```python
from build123d import *

# Parameters (mm, degrees)
SKETCH_1_R          = 2.5
EXTRUDE_1_DEPTH     = 2.5
EXTRUDE_1_2_DEPTH   = 2.5
EXTRUDE_1_3_DEPTH   = 2.5
SKETCH_2_R          = 1.5
EXTRUDE_2_DEPTH     = 2.5
SKETCH_3_W          = 5.060610533
SKETCH_3_H          = 13.613755096
EXTRUDE_3_DEPTH     = 2.5
SKETCH_4_W          = 80.650749302
SKETCH_4_H          = 55.377698756
EXTRUDE_4_DEPTH     = 2
SKETCH_5_W          = 80.650749302
SKETCH_5_H          = 55.377698756
SKETCH_5_W_2        = 75.650749302
SKETCH_5_H_2        = 50.377698756
EXTRUDE_5_DEPTH     = 13
FILLET_1_R          = 2.5
CUT_EXTRUDE_1_DEPTH = 2.6
SKETCH_8_W          = 3.315326588
SKETCH_8_H          = 13.986534041
CUT_EXTRUDE_2_DEPTH = 2
SKETCH_9_W          = 2.35
SKETCH_9_H          = 8.65
SKETCH_9_H_2        = 8.647957695
CUT_EXTRUDE_3_DEPTH = 3
FILLET_2_R          = 1
SKETCH_10_W         = 19.844488107
SKETCH_10_H         = 2.35
CUT_EXTRUDE_4_DEPTH = 3
FILLET_3_R          = 1
SKETCH_11_R         = 1.25
CUT_EXTRUDE_5_DEPTH = 6.8


with BuildPart() as part:
    # Sketch 1 → Extrude 1 (new body)
    with BuildSketch(Plane.XY):
        with Locations((-25.173975108, -5.08001016)):
            Circle(SKETCH_1_R)
    extrude(amount=EXTRUDE_1_DEPTH)



with BuildPart() as body_2:
    # Sketch 1 → Extrude 1 2 (new body)
    with BuildSketch(Plane.XY):
        with Locations((-25.173975108, -54.483108966)):
            Circle(SKETCH_1_R)
    extrude(amount=EXTRUDE_1_2_DEPTH)


with BuildPart() as body_3:
    # Sketch 1 → Extrude 1 3 (new body)
    with BuildSketch(Plane.XY):
        with Locations((27.94005588, -46.193418847)):
            Circle(SKETCH_1_R)
    extrude(amount=EXTRUDE_1_3_DEPTH)


with BuildPart() as part_1:
    add(part.part)

    add(body_2.part)  # Extrude 2 merges body 2

    add(body_3.part)  # Extrude 2 merges body 3
    # Sketch 2 → Extrude 2 (add)
    with BuildSketch(Plane(origin=(0, 0, 0), x_dir=(-1, 0, 0), z_dir=(0, 0, -1))):
        with Locations((25.173975108, -5.08001016)):
            Circle(SKETCH_2_R)
        with Locations((25.173975108, -54.483108966)):
            Circle(SKETCH_2_R)
        with Locations((-27.94005588, -46.193418847)):
            Circle(SKETCH_2_R)
    extrude(amount=EXTRUDE_2_DEPTH)



with BuildPart() as body_2_2:
    # Sketch 3 → Extrude 3 (new body)
    with BuildSketch(Plane(origin=(0, 0, 0), x_dir=(-1, 0, 0), z_dir=(0, 0, -1))):
        with Locations((-5.471223868, -19.889889862)):
            Rectangle(SKETCH_3_W, SKETCH_3_H)
    extrude(amount=-EXTRUDE_3_DEPTH)


with BuildPart() as part_2:
    add(part_1.part)

    add(body_2_2.part)  # Extrude 4 merges body 2 2
    # Sketch 4 → Extrude 4 (add)
    with BuildSketch(Plane.XY.offset(2.5)):
        with Locations((-9.398018796, -29.781559563)):
            Rectangle(SKETCH_4_W, SKETCH_4_H)
    extrude(amount=EXTRUDE_4_DEPTH)

    # Sketch 5 → Extrude 5 (add)
    with BuildSketch(Plane(origin=(0, 0, 2.5), x_dir=(-1, 0, 0), z_dir=(0, 0, -1))):
        with Locations((9.398018796, -29.781559563)):
            Rectangle(SKETCH_5_W, SKETCH_5_H)
        with Locations((9.398018796, -29.781559563)):
            Rectangle(SKETCH_5_W_2, SKETCH_5_H_2, mode=Mode.SUBTRACT)
    extrude(amount=EXTRUDE_5_DEPTH)

    # Fillet 1
    fillet_1_edges = [part_2.edges().sort_by_distance(p)[0] for p in [
        (-49.723393447, -2.092710185, -3),
        (-49.723393447, -57.470408941, -3),
        (30.927355855, -57.470408941, -3),
        (30.927355855, -2.092710185, -3),
    ]]
    fillet(fillet_1_edges, radius=FILLET_1_R)

    # Sketch 7 → Cut-Extrude 1 (cut)
    with BuildSketch(Plane.XZ.offset(57.470408941)):
        with BuildLine():
            Line((-1.675382515, -6.58006372), (-6.175382515, -6.58006372))
            ThreePointArc((-6.175382515, -6.58006372), (-9.675382515, -3.08006372), (-6.175382515, 0.41993628))
            Line((-6.175382515, 0.41993628), (-1.675382515, 0.41993628))
            ThreePointArc((-1.675382515, 0.41993628), (1.824617485, -3.08006372), (-1.675382515, -6.58006372))
        make_face()
    extrude(amount=-CUT_EXTRUDE_1_DEPTH, mode=Mode.SUBTRACT)

    # Sketch 8 → Cut-Extrude 2 (cut)
    with BuildSketch(Plane.XY.offset(4.5)):
        with Locations((15.823203351, -25.268606613)):
            Rectangle(SKETCH_8_W, SKETCH_8_H)
    extrude(amount=-CUT_EXTRUDE_2_DEPTH, mode=Mode.SUBTRACT)

    # Sketch 9 → Cut-Extrude 3 (cut)
    with BuildSketch(Plane(origin=(30.927355855, 0, 0), x_dir=(0, 0, -1), z_dir=(1, 0, 0))):
        with Locations((9.325, -10.033571247)):
            Rectangle(SKETCH_9_W, SKETCH_9_H)
        with Locations((9.325, -19.906568383)):
            Rectangle(SKETCH_9_W, SKETCH_9_H_2)
        with Locations((9.325, -29.718110236)):
            Rectangle(SKETCH_9_W, SKETCH_9_H)
    extrude(amount=-CUT_EXTRUDE_3_DEPTH, mode=Mode.SUBTRACT)

    # Fillet 2
    fillet_2_edges = [part_2.edges().sort_by_distance(p)[0] for p in [
        (29.677355855, -14.358571247, -8.15),
        (29.677355855, -5.708571247, -8.15),
        (29.677355855, -24.23054723, -8.15),
        (29.677355855, -15.582589535, -8.15),
        (29.677355855, -34.043110236, -8.15),
        (29.677355855, -25.393110236, -8.15),
    ]]
    fillet(fillet_2_edges, radius=FILLET_2_R)

    # Sketch 10 → Cut-Extrude 4 (cut)
    with BuildSketch(Plane(origin=(0, -2.092710185, 0), x_dir=(1, 0, 0), z_dir=(0, 1, 0))):
        with Locations((11.312306284, 9.325)):
            Rectangle(SKETCH_10_W, SKETCH_10_H)
    extrude(amount=-CUT_EXTRUDE_4_DEPTH, mode=Mode.SUBTRACT)

    # Fillet 3
    fillet_3_edges = [part_2.edges().sort_by_distance(p)[0] for p in [
        (21.234550337, -3.342710185, -8.15),
        (1.39006223, -3.342710185, -8.15),
    ]]
    fillet(fillet_3_edges, radius=FILLET_3_R)

    # Sketch 11 → Cut-Extrude 5 (cut)
    with BuildSketch(Plane.XZ.offset(57.470408941)):
        with Locations((-18.53025758, -6.91322852)):
            Circle(SKETCH_11_R)
    extrude(amount=-CUT_EXTRUDE_5_DEPTH, mode=Mode.SUBTRACT)


solid = part_2.part
```
Input: part model. Units: mm. Frame: model coordinates. A direction names the side the tool comes from. Round coordinates to 2 decimals unless told otherwise and drop trailing zeros. Loops run counter-clockwise (first coordinate to the right, second up) from the corner with the lowest first, then second, coordinate; pieces in that order, holes last. Notation, with made-up numbers: (7.5, -27) -> (42.5, -27) arc R29 ccw to (42.5, 10) -> close; hole circle Ø6 at (48, -12.5). An arc over 180 degrees is marked (long way). Use one line per item in the form item = value. Start each with the question number.
Item 1: Section query C-C on y = -38.5. Return the cut outline in (x, z).
Item 2: Section query A-A on y = -28. Return the cut outline in (x, z), then the cut area to 3 significant figures.
Item 3: Section query D-D on x = -21. Return the cut outline in (y, z), then the cut area to 3 significant figures.
Item 4: Mould query, pull axis Z, two halves, no side actions, for faces 1 (the face through (1.824, -56.238, -3.003)), 2 (the face through (2.941, -20, 1)), 3 (the face through (-10, -29, 2.5)). Classes: pulls with the +Z half, pulls with the -Z half, needs draft (parallel to the pull), parting line crosses it, or undercut.
Item 5: Section query B-B on x = 4.5. Return the cut outline in (y, z).
Item 6: Set-up query: faces 4 (the face through (16, -18.275, 4)), 5 (the face through (-9, -2.093, -3)), 6 (the face through (-25, -5, -2.5)), 7 (the face through (-4, -56, -6.58)). Return all of +Z, -Z, +X, -X, +Y, -Y with unobstructed straight access to the full face (end or side cutting, diameter ignored); none if empty.
Item 7: Material intervals for L1, parallel to X at y = -21.5, z = 0.25; L2, parallel to X at y = -54, z = -7.75; L3, parallel to Y at x = 27, z = -1, sorted ascending. Write a range as from..to.
Item 8: Contact query for flat-ended pins moving along their axis: pin 1 Ø0.7 at (x, z) = (29.5, -10) entering from +Y; pin 2 Ø3 at (x, y) = (30, -10) entering from -Z; pin 3 Ø1.1 at (x, z) = (29.5, -9.5) entering from +Y; pin 4 Ø1 at (x, y) = (28, -46.5) entering from -Z. Output: stop coordinate, or through.
Ans:
q1.outline = (-49.72, -10.5) -> (-47.22, -10.5) -> (-47.22, 2.5) -> (28.43, 2.5) -> (28.43, -10.5) -> (30.93, -10.5) -> (30.93, 4.5) -> (-49.72, 4.5) -> close
q2.outline = (-49.72, -10.5) -> (-47.22, -10.5) -> (-47.22, 2.5) -> (14.17, 2.5) -> (14.17, 4.5) -> (-49.72, 4.5) -> close; (17.48, 2.5) -> (28.43, 2.5) -> (28.43, -8.15) -> (30.93, -8.15) -> (30.93, 4.5) -> (17.48, 4.5) -> close
q2.area = 214 mm^2
q3.outline = (-57.47, -10.5) -> (-54.97, -10.5) -> (-54.97, 2.5) -> (-4.59, 2.5) -> (-4.59, -10.5) -> (-2.09, -10.5) -> (-2.09, 4.5) -> (-57.47, 4.5) -> close
q3.area = 176 mm^2
q4.face_1 = undercut
q4.face_2 = needs draft
q4.face_3 = pulls with the -Z half
q5.outline = (-57.47, -10.5) -> (-54.97, -10.5) -> (-54.97, 2.5) -> (-26.7, 2.5) -> (-26.7, 0) -> (-13.08, 0) -> (-13.08, 2.5) -> (-4.59, 2.5) -> (-4.59, -8.15) -> (-2.09, -8.15) -> (-2.09, 4.5) -> (-57.47, 4.5) -> close
q6.face_4 = +Z, -Z
q6.face_5 = +Z, -Z, +X, -X, +Y
q6.face_6 = -Z
q6.face_7 = -Y
q7.L1 = -49.72..-47.22, 2.94..8, 28.43..30.93
q7.L2 = -49.72..-47.22, 28.43..30.93
q7.L3 = -57.47..-54.97, -47.36..-45.02, -4.59..-2.09
q8.pin_1 = -2.2
q8.pin_2 = -8.15
q8.pin_3 = -2.15
q8.pin_4 = -10.5
